Check sheet for the modelled part. Datum: model origin and axes. Units: mm. A direction names the side the tool comes from. Round coordinates to 2 decimals unless told otherwise and drop trailing zeros. Write each loop counter-clockwise with the first axis right and the second up, starting at its lowest first coordinate (ties: lowest second). Pieces come first, ordered by that corner, then holes. Notation, with made-up numbers: M 3,-6 L 41,-6 A18 cw 41,21 Z; hole C -15.5,38 d11. An arc over 180 degrees is marked long. Answer in a Markdown table with one row per item.
Autodesk Inventor part; units mm, degrees
ref_plane "YZ Plane" through (0, 0, 0) normal (1, 0, 0) x (0, 1, 0)
ref_plane "XZ Plane" through (0, 0, 0) normal (0, 1, 0) x (-1, 0, 0)
ref_plane "XY Plane" through (0, 0, 0) normal (0, 0, 1) x (1, 0, 0)
sketch "草圖1" plane through (0, 0, 0) normal (0, 0, 1) x (1, 0, 0)
  arc A0 (-17.5, 0) -> (17.5, 0) centre (0, 0) ccw
  arc A1 (-20, 0) -> (20, 0) centre (0, 0) ccw
  line L0 (-20, 0) -> (-17.5, 0)
  line L1 (20, 0) -> (17.5, 0)
  line L2 (-35, 0) -> (35, 0)
  line L3 (-25, 0) -> (25, 0)
  line L4 (25, -60) -> (-25, -60)
  line L5 (-25, -60) -> (-25, 0)
  line L6 (-25, 0) -> (25, 0)
  line L7 (25, 0) -> (25, -60)
  line L8 (25, -60) -> (-25, 0) construction
  line L9 (-25, -60) -> (25, 0) construction
  line L10 (0, -72) -> (0, 12)
  point P0 (17.5, 0)
  point P1 (20, 0)
  point P2 (20, 0)
  point P3 (0, -30)
  dimension "d16" = 50
  dimension "d17" = 60
  dimension "d22" = 40
  dimension "d23" = 17.5
extrude "擠出1" add sketch "草圖1" along normal mid plane 20 contours L2 L10 A0 | A0 L10 A1 L0 | L10 L2 A0 | A0 L1 A1 L10
extrude "擠出2" add sketch "草圖1" along normal mid plane 5
sketch "草圖2" plane through (0, 0, 0) normal (1, 0, 0) x (0, 1, 0)
  line L0 (-10, -10) -> (-5, 10)
  line L1 (0, -2.5) -> (0, -10)
  line L2 (0, 10) -> (0, 2.5)
  line L3 (-20, -10) -> (0, -10)
  line L4 (0, 10) -> (-20, 10)
  point P0 (0, 0)
  dimension "d18" = 10
  dimension "d19" = 5
sketch "草圖3" plane through (0, 0, -10) normal (0, 0, -1) x (-1, 0, 0)
  arc A0 (-17.5, 0) -> (17.5, 0) centre (0, 0) ccw
  line L0 (25, 0) -> (-25, 0)
sweep "掃掠1" cut profiles "草圖3" path "草圖2" path curves L0
1. Section check B-B, the plane y = -19. Record the cut outline in (x, z) (3 decimals), and give its area (3 significant figures).
Found:
| item | result |
|---|---|
| outline | M -25,-2.5 L -6.245,-2.5 L -6.245,-10 L 6.245,-10 L 6.245,-2.5 L 25,-2.5 L 25,2.5 L 6.245,2.5 L 6.245,10 L -6.245,10 L -6.245,2.5 L -25,2.5 Z |
| area | 437 mm2 |
2. Scan lines: L1, parallel to Z at x = -14, y = -40; L2, parallel to X at y = -9, z = 3.5; L3, parallel to X at y = -4.5, z = -7.25. Record each from-to range of solid material in increasing order.
Found:
| item | result |
|---|---|
| L1 | z = -2.5 to 2.5 |
| L2 | x = -17.86 to -12.37, 12.37 to 17.86 |
| L3 | x = -19.49 to -16.71, 16.71 to 19.49 |
3. Access from +Z, -Z, +X, -X, +Y, -Y to the whole of each face (thin tool, end or side, straight path). Record for faces 1 (the face through (0, -20, 6)), 2 (the face through (0, -20, -6)), 3 (the face through (-25, -30, 0)).
Found:
| item | result |
|---|---|
| face 1 | +Z, -Y |
| face 2 | -Z, -Y |
| face 3 | +Z, -Z, -X, +Y, -Y |
4. Go/stop test with flat-tipped pins: pin 1 (1 mm diameter, centred on x = -17.5, y = -26, fed in from +Z); pin 2 (12 mm diameter, centred on x = -14.5, z = 4, fed in from -Y); pin 3 (6 mm diameter, centred on x = 0, z = -5, fed in from +Y). Record where each tip stops, or that it passes through.
Found:
| item | result |
|---|---|
| pin 1 | stops at z = 2.5 |
| pin 2 | stops at y = -60 |
| pin 3 | stops at y = -15.5 |
5. Section check A-A, the plane y = -51.5. Record the cut outline in (x, z).
Found:
| item | result |
|---|---|
| outline | M -25,-2.5 L 25,-2.5 L 25,2.5 L -25,2.5 Z |
